```python
from build123d import *

# Parameters (mm, degrees)
E_BAY_SHELL_R       = 41.275
E_BAY_SHELL_R_2     = 38.1
BOSS_EXTRUDE1_DEPTH = 203.2
LID_TOP_START       = -6.35
SKETCH2_R           = 38.1
SKETCH2_R_2         = 3.6195
SKETCH2_R_3         = 1.905
LID_TOP_DEPTH       = 6.35


with BuildPart() as part:
    # e-bay Shell → Boss-Extrude1 (new body)
    with BuildSketch(Plane.XY):
        Circle(E_BAY_SHELL_R)
        Circle(E_BAY_SHELL_R_2, mode=Mode.SUBTRACT)
    extrude(amount=BOSS_EXTRUDE1_DEPTH)

    # Sketch2 → lid-top (add)
    with BuildSketch(Plane.XY.offset(203.2).offset(LID_TOP_START)):
        Circle(SKETCH2_R)
        Circle(SKETCH2_R_2, mode=Mode.SUBTRACT)
        with Locations((-30.48, 0)):
            Circle(SKETCH2_R_2, mode=Mode.SUBTRACT)
        with Locations((21.231989214, 14.212140166)):
            Circle(SKETCH2_R_3, mode=Mode.SUBTRACT)
        with Locations(Location((30.48, 0, 0), (0, 0, 180))):
            Circle(SKETCH2_R_2, mode=Mode.SUBTRACT)
    lid_top = extrude(amount=LID_TOP_DEPTH)

    # Mirror3: lid-top across plane
    add(lid_top.mirror(Plane.XY.offset(101.6)))


solid = part.part
```
Design review of the part built by this model. Coordinates are the model's own, in mm. A direction names the side the tool comes from. Coordinates: 2 decimals unless noted, no trailing zeros. Order: outer loops, then holes, each group sorted by start corner. A loop starts at its lowest first (then second) coordinate and runs counter-clockwise, first axis right, second up. Notation, with made-up numbers: M 85.5,49 L 138.5,49 A15 cw 138.5,66 Z; hole C -6,67.25 d7. An arc over 180 degrees is marked long. Answer as a JSON object with one key per item and string values. Group by question number.
1) Tool access review of faces 4 (the flat face through (-1, -8, 196.85)), 5 (the cylindrical face through (19.83, 15.5, 3.22)): name each direction out of +Z, -Z, +X, -X, +Y, -Y from which nothing blocks a thin tool from reaching the whole face with its end or side.
2) For pin 1 (3 mm diameter, centred on y = -6.5, z = 144.5, fed in from -X); pin 2 (2 mm diameter, centred on y = -2.5, z = 107.5, fed in from +X); pin 3 (1.5 mm diameter, centred on y = -19.5, z = 56.5, fed in from +X); pin 4 (2 mm diameter, centred on x = -21, y = -29, fed in from -Z), all flat-tipped, find the tip position at first contact; note any pin that passes through.
3) Mouldability with a two-part tool opening along X and no side actions: class faces 1 (the cylindrical face through (-0.47, 3.59, 3.22)), 2 (the cylindrical face through (-8.948, -40.293, 100.178)), 3 (the flat face through (-1, -9, 0)) as pulls with the +X half, pulls with the -X half, needs draft (parallel to the pull), parting line crosses it, or undercut.
4) Wall thickness on L1, parallel to Z at x = -11, y = 8.5; L2, parallel to Y at x = 0, z = 144 (3 decimals); L3, parallel to X at y = 1.5, z = 110: over which ranges is each line inside the solid? List them lowest first.
5) Add section C-C, the plane y = 26. Write out the cut boundary in (x, z).
6) Add section D-D, the plane x = 9.5. Write out the cut boundary in (y, z), then the cut area to 3 significant figures.
7) Add section B-B, the plane y = 0. Count the separate pieces of the cut face and the enclosed holes in it, then the cut area to 3 significant figures.
Computed values:
{
 "1": {"face 4": "none", "face 5": "+Z, -Z"},
 "2": {"pin 1": "stops at x = -40.97", "pin 2": "stops at x = 41.25", "pin 3": "stops at x = 36.77", "pin 4": "stops at z = 0"},
 "3": {"face 1": "undercut", "face 2": "parting line crosses it", "face 3": "needs draft"},
 "4": {"L1": "z = 0 to 6.35, 196.85 to 203.2", "L2": "y = -41.275 to -38.1, 38.1 to 41.275", "L3": "x = -41.25 to -38.07, 38.07 to 41.25"},
 "5": {"outline": "M -32.06,0 L 32.06,0 L 32.06,203.2 L -32.06,203.2 Z; hole M -27.85,6.35 L 27.85,6.35 L 27.85,196.85 L -27.85,196.85 Z"},
 "6": {"outline": "M -40.17,0 L 40.17,0 L 40.17,203.2 L -40.17,203.2 Z; hole M -36.9,6.35 L 36.9,6.35 L 36.9,196.85 L -36.9,196.85 Z", "area": "2,270 mm^2"},
 "7": {"separate pieces": "6", "enclosed holes": "0", "area": "1,980 mm^2"}
}
